Part model, mm, in its own coordinate system. A direction names the side the tool comes from. Coordinates: 2 decimals unless noted, no trailing zeros. Order: outer loops, then holes, each group sorted by start corner. A loop starts at its lowest first (then second) coordinate and runs counter-clockwise, first axis right, second up.
1) Mould opens along Y. For faces 1 (the flat face through (-33.57, 36, 11.62)), 2 (the flat face through (-4.415, 22.019, 11.314)), 3 (the flat face through (0, -15, 12)) say: +Y half, -Y half, draft (parallel to the pull), parting line (faces both ways), or undercut.
2) Tool access for faces 4 (the cylindrical face through (-8.42, 27.22, 9.9)), 5 (the flat face through (-5, 12, 11)), 6 (the flat face through (-14, -21.471, 3)): list every direction of +Z, -Z, +X, -X, +Y, -Y with a clear straight run to the whole face (end or side of a thin tool).
3) Wall check: L1, parallel to Z at x = -2, y = -34; L2, parallel to X at y = -1, z = 10; L3, parallel to Z at x = -6.5, y = -37.5. Give the ranges that are in metal, low to high.
4) Cut at D-D (z = 19.5). List the corners of the cut face in (x, y), and give its area (3 significant figures).
5) Pin check, flat tips, straight feed: pin 1 Ø2.5 at (y, z) = (13.5, 11) entering from -X; pin 2 Ø0.8 at (x, z) = (-4.5, 11.5) entering from -Y; pin 3 Ø3 at (x, z) = (-19.5, 13) entering from +Y. Stop position of each tip, or through.
6) Cut at A-A (x = -22). List the corners of the cut face in (y, z), and give its area (3 significant figures).
7) Cut at B-B (y = -38). List the corners of the cut face in (x, z).
8) Cut at C-C (x = -9). List the corners of the cut face in (y, z), and give its area (3 significant figures).
```python
from build123d import *

# Parameters (mm, degrees)
ESQUISSE1_W             = 4
ESQUISSE1_H             = 85
BOSS_EXTRU_1_DEPTH      = 22.93
BOSS_EXTRU_5_DEPTH      = 22.95
CONG_1_R                = 2
ESQUISSE7_W             = 4
ESQUISSE7_H             = 21.820353027
BOSS_EXTRU_10_DEPTH     = 25.35
CONG_14_R               = 1
CONG_15_R               = 1
ESQUISSE9_R             = 1.8
ENL_V_MAT_EXTRU_1_DEPTH = 58
BOSS_EXTRU_11_DEPTH     = 1
BOSS_EXTRU_12_DEPTH     = 22.95


with BuildPart() as part:
    # Esquisse1 → Boss.-Extru.1 (new body)
    with BuildSketch(Plane.XY):
        with Locations((-2, -15.95097561)):
            Rectangle(ESQUISSE1_W, ESQUISSE1_H)
    extrude(amount=BOSS_EXTRU_1_DEPTH)

    # Esquisse2 → Boss.-Extru.5 (add)
    with BuildSketch(Plane.XY.offset(22.93)):
        Polygon((-32.681935281, 38.444276031), (0, 26.54902439), (0, 22.54902439), (-4, 22.54902439), (-34.435421614, 33.626611925), align=None)
    extrude(amount=-BOSS_EXTRU_5_DEPTH)

    # Congé1
    cong_1_edges = [part.edges().sort_by_distance(p)[0] for p in [
        (-2, -58.45097561, 22.93),
        (-2, -58.45097561, 0),
    ]]
    fillet(cong_1_edges, radius=CONG_1_R)

    # Esquisse7 → Boss.-Extru.10 (add)
    with BuildSketch(Plane(origin=(0, 0, 0), x_dir=(0, 0, -1), z_dir=(1, 0, 0))):
        with Locations((-2, -32.381152124)):
            Rectangle(ESQUISSE7_W, ESQUISSE7_H)
    extrude(amount=-BOSS_EXTRU_10_DEPTH)

    # Congé14
    cong_14_edges = [part.edges().sort_by_distance(p)[0] for p in [
        (-25.35, -43.291328637, 2),
        (-25.35, -21.47097561, 2),
    ]]
    fillet(cong_14_edges, radius=CONG_14_R)

    # Congé15
    cong_15_edges = [part.edges().sort_by_distance(p)[0] for p in [
        (-14.175, -43.291328637, 0),
        (-25.35, -32.381152123, 0),
        (-14.175, -21.47097561, 0),
        (-25.057106781, -21.763868829, 0),
        (-25.057106781, -42.998435418, 0),
    ]]
    fillet(cong_15_edges, radius=CONG_15_R)

    # Esquisse9 → Enlèv. mat.-Extru.1 (cut)
    with BuildSketch(Plane(origin=(0, 0, 0), x_dir=(1, 0, 0), z_dir=(0, 1, 0))):
        with Locations((-25.73017615, -11.416199304)):
            Circle(ESQUISSE9_R)
        with Locations((-9.38920851, -11.416199304)):
            Circle(ESQUISSE9_R)
    extrude(amount=ENL_V_MAT_EXTRU_1_DEPTH, mode=Mode.SUBTRACT)

    # Esquisse10 → Boss.-Extru.11 (add)
    with BuildSketch(Plane.ZY.offset(4)):
        Polygon((7.751431337, 10.464501792), (12.751431337, 10.464501792), (12.751431337, 15.464501792), (10.751431337, 15.464501792), (10.751431337, 12.464501792), (7.751431337, 12.464501792), align=None)
    extrude(amount=BOSS_EXTRU_11_DEPTH)

    # Esquisse13 → Boss.-Extru.12 (add)
    with BuildSketch(Plane.XY):
        Polygon((-5.151966744, 23.320636857), (-3.656231692, 20.681104413), (-2.075100003, 23.320636857), align=None)
    extrude(amount=BOSS_EXTRU_12_DEPTH)


solid = part.part
```
Geometry check:
1. face 1: +Y half
1. face 2: undercut
1. face 3: draft
2. face 4: +Y, -Y
2. face 5: +Z, -Z, -X, -Y
2. face 6: +Z, -Z, -X
3. L1: z = 0 to 22.93
3. L2: x = -4 to 0
3. L3: z = 0 to 4
4. outline: (-34.44, 33.63) - (-4.9, 22.88) - (-4, 21.29) - (-4, -58.45) - (0, -58.45) - (0, 26.55) - (-32.68, 38.44) - close
4. area: 505 mm2
5. pin 1: stops at x = -5
5. pin 2: stops at y = 10.46
5. pin 3: stops at y = 34.19
6. outline: (-43.29, 1) arc R1 ccw to (-42.29, 0) - (-22.47, 0) arc R1 ccw to (-21.47, 1) - (-21.47, 4) - (-43.29, 4) - close; (29.1, -0.02) - (34.56, -0.02) - (34.56, 22.93) - (29.1, 22.93) - close
6. area: 212 mm2
7. outline: (-25.35, 1) arc R1 ccw to (-24.35, 0) - (0, 0) - (0, 22.93) - (-4, 22.93) - (-4, 4) - (-25.35, 4) - close
8. outline: (-43.29, 1) arc R1 ccw to (-42.29, 0) - (-22.47, 0) arc R1 ccw to (-21.47, 1) - (-21.47, 4) - (-43.29, 4) - close; (24.37, -0.02) - (29.82, -0.02) - (29.82, 9.66) - (24.37, 9.66) - close; (24.37, 13.17) - (29.82, 13.17) - (29.82, 22.93) - (24.37, 22.93) - close
8. area: 193 mm2
